from build123d import *

# Parameters (mm, degrees)
ESQUISSE1_W          = 6
ESQUISSE1_H          = 20
BOSS_EXTRU_2_DEPTH   = 6
ESQUISSE1_W_2        = 16
ESQUISSE1_H_2        = 6
BOSS_EXTRU_2_2_DEPTH = 6
BOSS_EXTRU_2_3_DEPTH = 6
BOSS_EXTRU_2_4_DEPTH = 6
BOSS_EXTRU_3_DEPTH   = 16


with BuildPart() as part:
    # Esquisse1 → Boss.-Extru.2 (new body)
    with BuildSketch(Plane.ZY.offset(97.003078089)):
        with Locations((181.00005, -2.704155421)):
            Rectangle(ESQUISSE1_W, ESQUISSE1_H)
    extrude(amount=BOSS_EXTRU_2_DEPTH)



with BuildPart() as body_2:
    # Esquisse1 → Boss.-Extru.2 2 (new body)
    with BuildSketch(Plane.ZY.offset(97.003078089)):
        with Locations((192.00005, 25.295844579)):
            Rectangle(ESQUISSE1_W_2, ESQUISSE1_H_2)
    extrude(amount=BOSS_EXTRU_2_2_DEPTH)


with BuildPart() as body_3:
    # Esquisse1 → Boss.-Extru.2 3 (new body)
    with BuildSketch(Plane.ZY.offset(97.003078089)):
        with Locations((203.00005, -2.704155421)):
            Rectangle(ESQUISSE1_W, ESQUISSE1_H)
    extrude(amount=BOSS_EXTRU_2_3_DEPTH)


with BuildPart() as body_4:
    # Esquisse1 → Boss.-Extru.2 4 (new body)
    with BuildSketch(Plane.ZY.offset(97.003078089)):
        with Locations((192.00005, -30.704155421)):
            Rectangle(ESQUISSE1_W_2, ESQUISSE1_H_2)
    extrude(amount=BOSS_EXTRU_2_4_DEPTH)


with BuildPart() as part_1:
    add(part.part)

    add(body_2.part)  # Boss.-Extru.3 merges body 2

    add(body_3.part)  # Boss.-Extru.3 merges body 3

    add(body_4.part)  # Boss.-Extru.3 merges body 4
    # Esquisse2 → Boss.-Extru.3 (add)
    with BuildSketch(Plane(origin=(0, 0, 200.00005), x_dir=(-1, 0, 0), z_dir=(0, 0, -1))):
        Polygon((103.003078089, 22.295844579), (97.003078089, 22.295844579), (97.003078089, 7.295844579), (97.003078089, -12.704155421), (97.003078089, -27.704155421), (103.003078089, -27.704155421), (103.003078089, -12.704155421), (103.003078089, 7.295844579), align=None)
    extrude(amount=BOSS_EXTRU_3_DEPTH)


solid = part_1.part
Geometry check sheet. Reference: the model listing, model coordinates, mm. A direction names the side the tool comes from. Round coordinates to 2 decimals unless told otherwise and drop trailing zeros. Write each loop counter-clockwise with the first axis right and the second up, starting at its lowest first coordinate (ties: lowest second). Pieces come first, ordered by that corner, then holes. Notation, with made-up numbers: (-29.5, 71) -> (-10.5, 71) arc R17 cw to (-10.5, 97) -> close; hole circle Ø10 at (50, -19.5). An arc over 180 degrees is marked (long way). One line per item, written item: value. Start each with the question number.
(1) Go/stop test with flat-tipped pins: pin 1 Ø3 at (x, z) = (-100.5, 180) entering from +Y; pin 2 Ø2 at (x, y) = (-102, 21) entering from +Z; pin 3 Ø1.8 at (x, y) = (-100, -25) entering from -Z. Record where each tip stops, or that it passes through.
(2) Cross-section at A-A, the plane x = -98.75. Record the cut outline in (y, z), and give its area (3 significant figures).
(3) Cross-section at C-C, the plane z = 202.5. Record the cut outline in (x, y).
(4) Scan lines: line 1 (Z direction, x = -99.6, y = -29); line 2 (Y direction, x = -99.7, z = 203.25). Record each from-to range of solid material in increasing order. Write a range as [from, to].
(5) Access from +Z, -Z, +X, -X, +Y, -Y to the whole of each face (thin tool, end or side, straight path). Record for faces 1 (the flat face through (-100, 18, 200)), 2 (the flat face through (-100, -23, 184)), 3 (the flat face through (-100, -12.704, 203)), 4 (the flat face through (-100, 18, 184)).
(6) Cross-section at B-B, the plane y = 11. Record the cut outline in (x, z).
Answer:
1. pin 1: y = 7.3
1. pin 2: z = 200
1. pin 3: z = 184
2. outline: (-33.7, 184) -> (-12.7, 184) -> (-12.7, 178) -> (7.3, 178) -> (7.3, 184) -> (28.3, 184) -> (28.3, 200) -> (7.3, 200) -> (7.3, 206) -> (-12.7, 206) -> (-12.7, 200) -> (-33.7, 200) -> close
2. area: 1,230 mm²
3. outline: (-103, -12.7) -> (-97, -12.7) -> (-97, 7.3) -> (-103, 7.3) -> close
4. line 1: [184, 200]
4. line 2: [-12.7, 7.3]
5. face 1: +Z, +X, -X, +Y
5. face 2: -Z, +X, -X, -Y
5. face 3: +Z, +X, -X, -Y
5. face 4: -Z, +X, -X, +Y
6. outline: (-103, 184) -> (-97, 184) -> (-97, 200) -> (-103, 200) -> close
